Verification items for this drawing (mm, ordinates from the low corner). Round coordinates to 2 decimals unless told otherwise and drop trailing zeros. Loops run counter-clockwise (first coordinate to the right, second up) from the corner with the lowest first, then second, coordinate; pieces in that order, holes last. Notation, with made-up numbers: (7.25, 30.5) - (57.25, 30.5) arc R25 cw to (57.25, 55.5) - close; hole circle Ø11 at (89, 66). An arc over 180 degrees is marked (long way). Answer in a Markdown table with one row per item. Add a question column.
(1) Cross-section at B-B on x = 3. Enter the section's corners in (y, z), then the cut area to 3 significant figures.
(2) Mould release check, pull along X, two halves, no side actions. Record for the marked faces 1, 2 and 3: +X half, -X half, draft (parallel to the pull), parting line (faces both ways), or undercut.
(3) Cross-section at D-D on z = 0.8. Enter the section's corners in (x, y).
(4) Cross-section at C-C on y = 12.25. Enter the section's corners in (x, z).
(5) Thickness scan on line 1 along X through (y, z) = (16.25, 1.75); line 2 along Y through (x, z) = (27, 2.35); line 3 along X through (y, z) = (16.75, 2.8). Record the ranges inside material, lowest first.
(6) Cross-section at A-A on y = 27. Enter the section's corners in (x, z).
(7) Gauge pin test, flat ends, axial feed: pin 1 (17.5 mm diameter, centred on x = 16, y = 8.5, fed in from +Z); pin 2 (0.6 mm diameter, centred on x = 15.5, z = 3, fed in from -Y); pin 3 (1.2 mm diameter, centred on x = 27, y = 27, fed in from +Z); pin 4 (0.8 mm diameter, centred on x = 10.5, z = 1.5, fed in from -Y). Record the tip position at first contact, or that the pin passes through.
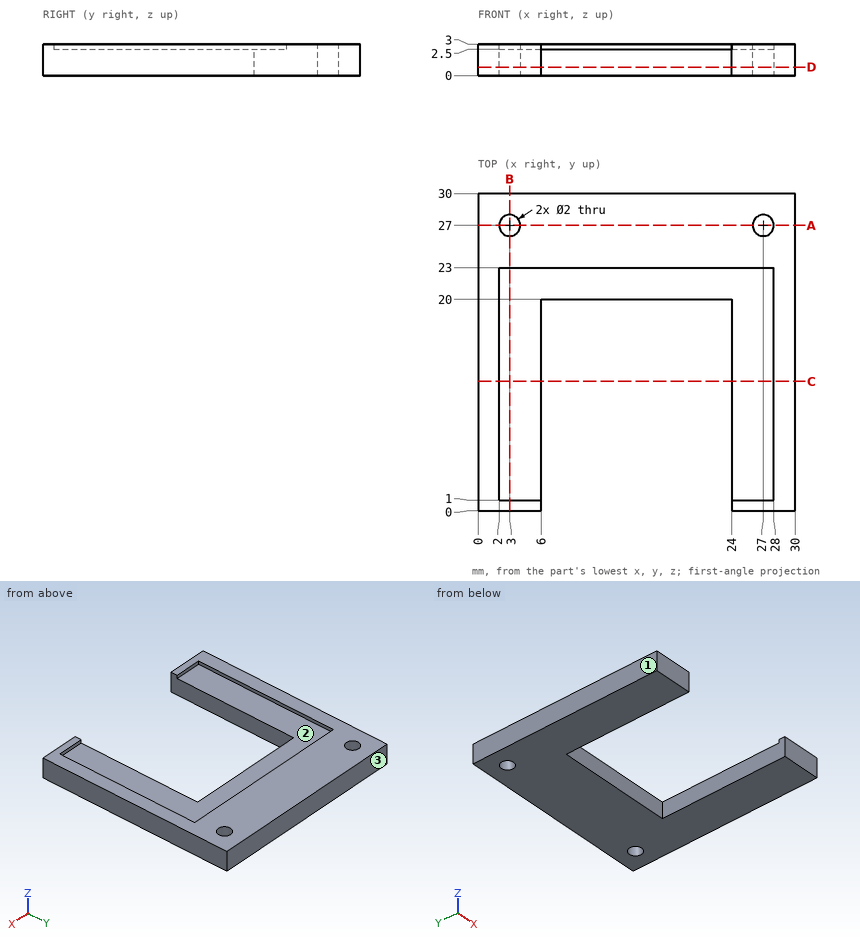
Answers:
| question | item | result |
|---|---|---|
| 1 | outline | (0, 0) - (26, 0) - (26, 3) - (23, 3) - (23, 2.5) - (1, 2.5) - (1, 3) - (0, 3) - close; (28, 0) - (30, 0) - (30, 3) - (28, 3) - close |
| 1 | area | 73.0 mm^2 |
| 2 | face 1 | -X half |
| 2 | face 2 | undercut |
| 2 | face 3 | draft |
| 3 | outline | (0, 0) - (6, 0) - (6, 20) - (24, 20) - (24, 0) - (30, 0) - (30, 30) - (0, 30) - close; hole circle Ø2 at (3, 27); hole circle Ø2 at (27, 27) |
| 4 | outline | (0, 0) - (6, 0) - (6, 2.5) - (2, 2.5) - (2, 3) - (0, 3) - close; (24, 0) - (30, 0) - (30, 3) - (28, 3) - (28, 2.5) - (24, 2.5) - close |
| 5 | line 1 | x = 0 to 6, 24 to 30 |
| 5 | line 2 | y = 0 to 26, 28 to 30 |
| 5 | line 3 | x = 0 to 2, 28 to 30 |
| 6 | outline | (0, 0) - (2, 0) - (2, 3) - (0, 3) - close; (4, 0) - (26, 0) - (26, 3) - (4, 3) - close; (28, 0) - (30, 0) - (30, 3) - (28, 3) - close |
| 7 | pin 1 | stops at z = 2.5 |
| 7 | pin 2 | stops at y = 23 |
| 7 | pin 3 | passes through |
| 7 | pin 4 | stops at y = 20 |
